Could you check a few things on this model? Use its own coordinates, in mm. Coordinates: 2 decimals unless noted, no trailing zeros. Write each loop counter-clockwise with the first axis right and the second up, starting at its lowest first coordinate (ties: lowest second). Pieces come first, ordered by that corner, then holes.
```python
from build123d import *

# Parameters (mm, degrees)
SKETCH002_W     = 1.651
SKETCH002_H     = 7.62
PAD_DEPTH       = 2.54
SKETCH003_W     = 0.761982
SKETCH003_H     = 0.762
SKETCH003_W_2   = 0.761985
SKETCH003_W_3   = 0.761994
POCKET_DEPTH    = 1.778
SKETCH004_R     = 0.381
POCKET001_DEPTH = 1.652


with BuildPart() as part:
    # Sketch002 → Pad (new body)
    with BuildSketch(Plane.YZ):
        with Locations((0.8255, 0)):
            Rectangle(SKETCH002_W, SKETCH002_H)
    extrude(amount=PAD_DEPTH)

    # Sketch003 (on Face6 of Pad) → Pocket (cut)
    with BuildSketch(Plane.YZ.offset(2.54)):
        with Locations((1.27001, 2.54)):
            Rectangle(SKETCH003_W, SKETCH003_H)
        with Locations((1.270008, 0)):
            Rectangle(SKETCH003_W_2, SKETCH003_H)
        with Locations((1.270004, -2.54)):
            Rectangle(SKETCH003_W_3, SKETCH003_H)
    extrude(amount=-POCKET_DEPTH, mode=Mode.SUBTRACT)

    # Sketch004 (on Face2 of Pocket) → Pocket001 (cut, through all)
    with BuildSketch(Plane(origin=(0, 0, 0), x_dir=(0, 0, -1), z_dir=(0, -1, 0))):
        with Locations((0, 1.27)):
            Circle(SKETCH004_R)
        with Locations((-2.54, 1.27)):
            Circle(SKETCH004_R)
        with Locations((2.54, 1.27)):
            Circle(SKETCH004_R)
    extrude(amount=-POCKET001_DEPTH, mode=Mode.SUBTRACT)


solid = part.part
```
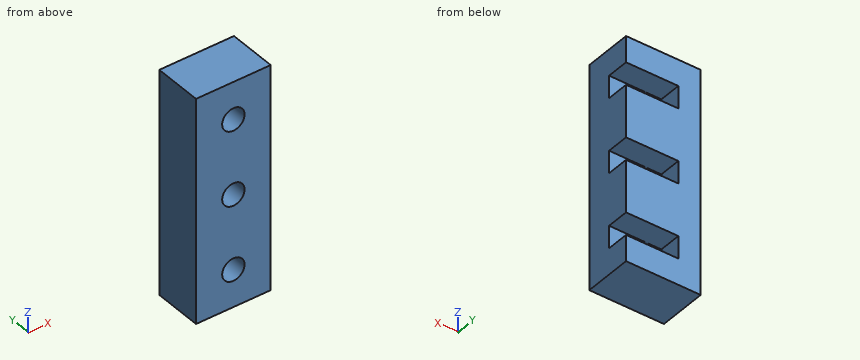
1. I want a section at C-C on x = 1.35. Give the number of separate pieces and of enclosed holes in the cut face, plus the area to 3 significant figures.
Verdict:
separate pieces: 4
enclosed holes: 0
area: 8.85 mm2
2. Please list where these lines run through material, in increasing order: line 1 along Z through (x, y) = (1.27, 0.7); line 2 along X through (y, z) = (0.6, 0).
Verdict:
line 1: z = -3.81 to -2.92, -2.16 to -0.38, 0.38 to 2.16, 2.92 to 3.81
line 2: x = 0 to 0.89, 1.65 to 2.54
3. I want a section at B-B on y = 1.15. Please give me the cut outline in (x, z).
Verdict:
outline: (0, -3.81) - (2.54, -3.81) - (2.54, -2.92) - (0.76, -2.92) - (0.76, -2.16) - (2.54, -2.16) - (2.54, -0.38) - (0.76, -0.38) - (0.76, 0.38) - (2.54, 0.38) - (2.54, 2.16) - (0.76, 2.16) - (0.76, 2.92) - (2.54, 2.92) - (2.54, 3.81) - (0, 3.81) - close
4. I want a section at D-D on y = 0.75. Please give me the cut outline in (x, z).
Verdict:
outline: (0, -3.81) - (2.54, -3.81) - (2.54, 3.81) - (0, 3.81) - close; hole circle Ø0.76 at (1.27, -2.54); hole circle Ø0.76 at (1.27, 0); hole circle Ø0.76 at (1.27, 2.54)
5. I want a section at A-A on z = 2.54. Please give me the cut outline in (x, y), plus the area to 3 significant figures.
Verdict:
outline: (0, 0) - (0.89, 0) - (0.89, 0.89) - (0.76, 0.89) - (0.76, 1.65) - (0, 1.65) - close; (1.65, 0) - (2.54, 0) - (2.54, 0.89) - (1.65, 0.89) - close
area: 2.16 mm2
6. For pin 1 (0.6 mm diameter, centred on x = 2, z = 0, fed in from +Y), with a flat end and sliding along its axis, tell me the tip position at first contact or that it passes through.
Verdict:
pin 1: stops at y = 0.89
